from build123d import *

# Parameters (mm, degrees)
F1_DEPTH = 0.5


with BuildPart() as f1:
    # F0 (on Top) → F1 (new body)
    with BuildSketch(Plane.XY):
        with BuildLine():
            Line((-5.81324, -4.248087), (-8.1605, -4.248087))
            Line((-8.1605, -4.248087), (-10.732831, -5.587158))
            ThreePointArc((-10.732831, -5.587158), (-10.68629, -5.675668), (-10.639018, -5.763791))
            Line((-10.639018, -5.763791), (-9.031771, -6.233106))
            ThreePointArc((-9.031771, -6.233106), (-8.681479, -6.615756), (-8.859146, -7.103157))
            Line((-8.859146, -7.103157), (-9.440273, -7.569098))
            ThreePointArc((-9.440273, -7.569098), (-9.377396, -7.646858), (-9.313879, -7.724096))
            Line((-9.313879, -7.724096), (-7.646027, -7.871644))
            ThreePointArc((-7.646027, -7.871644), (-7.227963, -8.178805), (-7.307377, -8.691464))
            Line((-7.307377, -8.691464), (-7.786714, -9.261592))
            ThreePointArc((-7.786714, -9.261592), (-7.709906, -9.325629), (-7.632571, -9.389028))
            Line((-7.632571, -9.389028), (-5.967894, -9.209166))
            ThreePointArc((-5.967894, -9.209166), (-5.498046, -9.429093), (-5.476171, -9.947405))
            Line((-5.476171, -9.947405), (-5.835387, -10.599918))
            ThreePointArc((-5.835387, -10.599918), (-5.747585, -10.647782), (-5.659391, -10.694919))
            Line((-5.659391, -10.694919), (-4.061547, -10.194525))
            ThreePointArc((-4.061547, -10.194525), (-3.55788, -10.318807), (-3.435553, -10.822952))
            Line((-3.435553, -10.822952), (-3.660912, -11.532897))
            ThreePointArc((-3.660912, -11.532897), (-3.565474, -11.562759), (-3.469792, -11.591831))
            Line((-3.469792, -11.591831), (-1.999883, -10.790041))
            ThreePointArc((-1.999883, -10.790041), (-1.48166, -10.813925), (-1.263558, -11.284624))
            Line((-1.263558, -11.284624), (-1.346442, -12.024853))
            ThreePointArc((-1.346442, -12.024853), (-1.247017, -12.03557), (-1.147507, -12.045465))
            Line((-1.147507, -12.045465), (0.138257, -10.972939))
            ThreePointArc((0.138257, -10.972939), (0.651219, -10.895513), (0.956757, -11.314766))
            Line((0.956757, -11.314766), (1.019517, -12.056973))
            ThreePointArc((1.019517, -12.056973), (1.119126, -12.048135), (1.218659, -12.038475))
            Line((1.218659, -12.038475), (2.271109, -10.736227))
            ThreePointArc((2.271109, -10.736227), (2.759196, -10.560452), (3.140484, -10.912226))
            Line((3.140484, -10.912226), (3.346488, -11.628027))
            ThreePointArc((3.346488, -11.628027), (3.442474, -11.599973), (3.538224, -11.571127))
            Line((3.538224, -11.571127), (4.317114, -10.088956))
            ThreePointArc((4.317114, -10.088956), (4.76166, -9.821553), (5.204118, -10.092396))
            Line((5.204118, -10.092396), (5.545489, -10.75442))
            ThreePointArc((5.545489, -10.75442), (5.634179, -10.708222), (5.722484, -10.661293))
            Line((5.722484, -10.661293), (6.19803, -9.055879))
            ThreePointArc((6.19803, -9.055879), (6.582035, -8.707073), (7.068744, -8.886629))
            Line((7.068744, -8.886629), (7.532427, -9.469559))
            ThreePointArc((7.532427, -9.469559), (7.610431, -9.406984), (7.687914, -9.343766))
            Line((7.687914, -9.343766), (7.833117, -7.579728))
            ThreePointArc((7.833117, -7.579728), (8.509339, -6.811839), (9.110578, -5.983926))
            ThreePointArc((9.110578, -5.983926), (9.242449, -5.18285), (8.736494, -4.547931))
            Line((8.736494, -4.547931), (8.1605, -4.248087))
            Line((8.1605, -4.248087), (5.81324, -4.248087))
            ThreePointArc((5.81324, -4.248087), (5.678957, -4.425997), (5.539231, -4.599665))
            Line((5.539231, -4.599665), (6.59, -6.41965))
            ThreePointArc((6.59, -6.41965), (5.83151, -7.115722), (5, -7.722694))
            Line((5, -7.722694), (5, -7.822694))
            ThreePointArc((5, -7.822694), (0, -9.284101), (-5, -7.822694))
            Line((-5, -7.822694), (-5, -7.722694))
            ThreePointArc((-5, -7.722694), (-5.83151, -7.115722), (-6.59, -6.41965))
            Line((-6.59, -6.41965), (-5.539231, -4.599665))
            ThreePointArc((-5.539231, -4.599665), (-5.678957, -4.425997), (-5.81324, -4.248087))
        make_face()
    extrude(amount=F1_DEPTH)


solid = f1.part
Work out the finished part from the listing and answer in its coordinate system (mm). A direction names the side the tool comes from. Round coordinates to 2 decimals unless told otherwise and drop trailing zeros. Loops run counter-clockwise (first coordinate to the right, second up) from the corner with the lowest first, then second, coordinate; pieces in that order, holes last. Notation, with made-up numbers: (-17, 76.25) -> (29, 76.25) arc R9 cw to (29, 90.25) -> close; hole circle Ø11 at (-40, 28). An arc over 180 degrees is marked (long way). Use one line per item in the form item = value.
(1) Find section A-A on y = -6.75. Give the vertices of the cut face in (x, z).
Answer list:
outline = (-8.67, 0) -> (-6.25, 0) -> (-6.25, 0.5) -> (-8.67, 0.5) -> close; (6.25, 0) -> (8.56, 0) -> (8.56, 0.5) -> (6.25, 0.5) -> close
(2) Find section B-B on x = -2.25. Give the vertices of the cut face in (y, z), then the cut area to 3 significant figures.
Answer list:
outline = (-10.93, 0) -> (-9.01, 0) -> (-9.01, 0.5) -> (-10.93, 0.5) -> close
area = 0.960 mm2
(3) A flat-ended cylindrical pin translates along its axis: P1, Ø2, axis at x = -2.5, y = -10.5, coming from the -Z side. Find the tip coordinate at first contact, or state that the pin passes through.
Answer list:
P1 = 0
(4) Straight lines are drawn through the part: line 1 (X direction, y = -11.5, z = 0.3); line 2 (X direction, y = -8.5, z = 0.45); line 3 (X direction, y = -5, z = 0.3). For each, find the intervals that lie inside material, in ascending order.
Answer list:
line_1 = -3.65 to -3.3, -1.29 to -0.49, 0.97 to 1.65, 3.31 to 3.58
line_2 = -7.21 to -3.73, 3.73 to 7.76
line_3 = -9.6 to -5.77, 5.77 to 9.18
(5) A tool of negligible diameter and unlimited length cuts with its end or side. For faces 1 (the flat face through (-6.07, -5.52, 0.25)), 2 (the flat face through (-0.514, -11.517, 0.246)), 3 (the cylindrical face through (8.5, -6.823, 0.246)), from which of +Z, -Z, +X, -X, +Y, -Y can it reach the whole face along a straight path? Write none if from no direction.
Answer list:
face_1 = +Z, -Z
face_2 = +Z, -Z, -Y
face_3 = +Z, -Z, +X, -Y
(6) Find section D-D on x = 0.5. Give the vertices of the cut face in (y, z), then the cut area to 3 significant figures.
Answer list:
outline = (-10.86, 0) -> (-9.27, 0) -> (-9.27, 0.5) -> (-10.86, 0.5) -> close
area = 0.794 mm2
(7) For a pull along Y with two mould halves and no side action, classify faces 4 (the cylindrical face through (-5.82, -7.125, 0.246)), 5 (the flat face through (-2.75, -11.2, 0.25)), 6 (the cylindrical face through (0.074, -9.284, 0.246)) as released by +Y, released by -Y, zero draft, split by the parting line, or undercut.
Answer list:
face_4 = undercut
face_5 = released by -Y
face_6 = released by +Y
(8) Find section C-C on y = -8.25. Give the vertices of the cut face in (x, z).
Answer list:
outline = (-7.2, 0) -> (-4.26, 0) -> (-4.26, 0.5) -> (-7.2, 0.5) -> close; (4.26, 0) -> (7.78, 0) -> (7.78, 0.5) -> (4.26, 0.5) -> close
